Geometry check sheet. Reference: the model listing, model coordinates, mm. A direction names the side the tool comes from. Give positions to 0.01 mm unless a question says otherwise; leave off trailing zeros. Order: outer loops, then holes, each group sorted by start corner. A loop starts at its lowest first (then second) coordinate and runs counter-clockwise, first axis right, second up. Notation, with made-up numbers: M -3,51 L 22,51 A11 cw 22,60 Z; hole C 76.25,-16.5 d10. An arc over 180 degrees is marked long. Answer as CSV lines item,"result".
from build123d import *

# Parameters (mm, degrees)
F0_W      = 100
F0_H      = 100
F1_DEPTH  = 100
F2_W      = 100
F2_H      = 75
F3_DEPTH  = 100.001
F4_R      = 25
F5_DEPTH  = 17
F7_DEPTH  = 92
F8_W      = 30.7691868506
F8_H      = 32.9230235268
F9_DEPTH  = 100.001
F11_DEPTH = 30


with BuildPart() as f1:
    # F0 (on Front) → F1 (new body)
    with BuildSketch(Plane.XZ):
        with Locations((50, 50)):
            Rectangle(F0_W, F0_H)
    extrude(amount=-F1_DEPTH)

    # F2 (on face) → F3 (cut, through all)
    with BuildSketch(Plane.YZ.offset(100)):
        with Locations((50, 62.5)):
            Rectangle(F2_W, F2_H)
    extrude(amount=-F3_DEPTH, mode=Mode.SUBTRACT)

    # F4 (on face) → F5 (cut)
    with BuildSketch(Plane.XY.offset(25)):
        with Locations((40, 60)):
            Circle(F4_R)
    extrude(amount=-F5_DEPTH, mode=Mode.SUBTRACT)

    # F6 (on face) → F7 (join)
    with BuildSketch(Plane.XY.offset(8)):
        with BuildLine():
            Line((30, 37.0871215252), (30, 82.9128784748))
            ThreePointArc((30, 82.9128784748), (15, 60), (30, 37.0871215252))
        make_face()
        with BuildLine():
            Line((62.9128784748, 50), (45, 50))
            Line((45, 50), (45, 35.5051025722))
            ThreePointArc((45, 35.5051025722), (55.7260201274, 40.5656929387), (62.9128784748, 50))
        make_face()
    extrude(amount=F7_DEPTH)

    # F8 (on face) → F9 (cut, through all)
    with BuildSketch(Plane.XZ):
        with Locations((54.3266609311, 101.4615117634)):
            Rectangle(F8_W, F8_H)
    extrude(amount=-F9_DEPTH, mode=Mode.SUBTRACT)

    # F10 (on face) → F11 (cut)
    with BuildSketch(Plane.YZ.offset(100)):
        Polygon((40.9007441433, 0), (50, 25), (0, 25), (0, 0), align=None)
    extrude(amount=-F11_DEPTH, mode=Mode.SUBTRACT)


solid = f1.part
(1) Section check C-C on y = 59. Enter the section's corners in (x, z), then the cut area to 3 significant figures.
The answers:
outline,"M 0,0 L 100,0 L 100,25 L 64.98,25 L 64.98,8 L 30,8 L 30,100 L 15.02,100 L 15.02,25 L 0,25 Z"
area,"3,030 mm2"
(2) Draft check along X on faces 1 (the face through (0, 49, 12)), 2 (the face through (37.27, 35.15, 16.62)), 3 (the face through (57.97, 77.38, 16.62)), 4 (the face through (55.595, 40.461, 54.58)). Enter one of: +X half, -X half, draft (parallel to the pull), parting line (faces both ways), or undercut.
The answers:
face 1,"-X half"
face 2,"undercut"
face 3,"undercut"
face 4,"+X half"
(3) Section check D-D on z = 10. Enter the section's corners in (x, y).
The answers:
outline,"M 0,0 L 70,0 L 70,44.54 L 100,44.54 L 100,100 L 0,100 Z; hole M 30,37.09 A25 ccw 45,35.51 L 45,50 L 62.91,50 A25 ccw 30,82.91 Z"
(4) Section check B-B on x = 20. Enter the section's corners in (y, z).
The answers:
outline,"M 0,0 L 100,0 L 100,25 L 75,25 L 75,100 L 45,100 L 45,25 L 0,25 Z"
(5) Section check A-A on z = 48. Enter the section's corners in (x, y), then the cut area to 3 significant figures.
The answers:
outline,"M 30,37.09 L 30,82.91 A25 ccw Z; M 45,35.51 A25 ccw 62.91,50 L 45,50 Z"
area,"669 mm2"
(6) Gauge pin test, flat ends, axial feed: P1, Ø2, axis at x = 86.5, z = 25, coming from the -Y side; P2, Ø17.5, axis at x = 53, y = 56.5, coming from the +Z side; P3, Ø20, axis at y = 17, z = 18, coming from the +X side. Record the tip position at first contact, or that the pin passes through.
The answers:
P1,"stops at y = 49.64"
P2,"stops at z = 85"
P3,"stops at x = 70"
(7) Tool access check on faces 5 (the face through (15, 60, 62)), 6 (the face through (100, 70, 12)), 7 (the face through (45, 43, 46)), 8 (the face through (52, 44, 85)), 9 (the face through (70, 25, 13)). Record the directions out of +Z, -Z, +X, -X, +Y, -Y that give a thin tool (end or side, any length) a straight path to the whole face; none if there is none.
The answers:
face 5,"+Z, -X"
face 6,"+Z, -Z, +X, +Y, -Y"
face 7,"+Z"
face 8,"+Z, +X, +Y, -Y"
face 9,"+Z, +X, -Y"
(8) Material ranges on line 1 (X direction, y = 39, z = 16); line 2 (Z direction, x = 60, y = 13); line 3 (Z direction, x = 36, y = 66), recorded low to high.
The answers:
line 1,"x = 0 to 30, 45 to 70"
line 2,"z = 0 to 25"
line 3,"z = 0 to 8"
